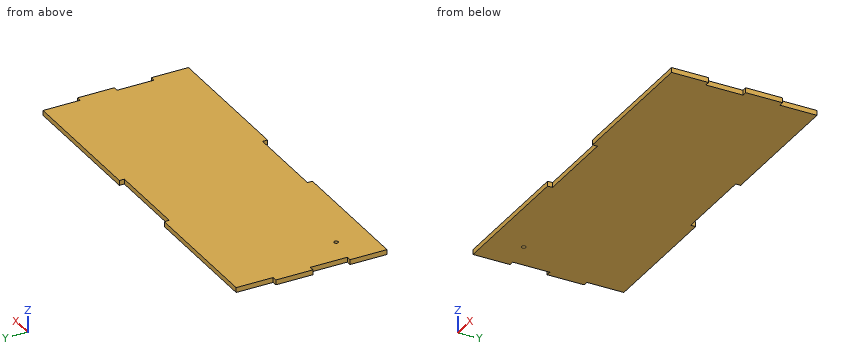
```python
from build123d import *

# Parameters (mm, degrees)
SKETCH1_R           = 1.25
BOSS_EXTRUDE1_DEPTH = 3


with BuildPart() as part:
    # Sketch1 → Boss-Extrude1 (new body)
    with BuildSketch(Plane.XY):
        Polygon((-2, 47), (78, 47), (78, 44), (128, 44), (128, 47), (213, 47), (213, 24.5), (216, 24.5), (216, 2), (213, 2), (213, -20.5), (216, -20.5), (216, -43), (213, -43), (128, -43), (128, -40), (78, -40), (78, -43), (-2, -43), (-5, -43), (-5, -20.5), (-2, -20.5), (-2, 2), (-5, 2), (-5, 24.5), (-2, 24.5), align=None)
        with Locations((15, -23)):
            Circle(SKETCH1_R, mode=Mode.SUBTRACT)
    extrude(amount=BOSS_EXTRUDE1_DEPTH)


solid = part.part
```
Check sheet for the modelled part. Datum: model origin and axes. Units: mm. Round coordinates to 2 decimals unless told otherwise and drop trailing zeros. Loops run counter-clockwise (first coordinate to the right, second up) from the corner with the lowest first, then second, coordinate; pieces in that order, holes last. Notation, with made-up numbers: (-9.75, -36.75) -> (35.25, -36.75) arc R20 ccw to (35.25, -16.75) -> close; hole circle Ø2 at (11.25, 40). An arc over 180 degrees is marked (long way). Write item = value, one per line. Start each with the question number.
1) Gauge pin test, flat ends, axial feed: pin 1 Ø0.9 at (y, z) = (45.5, 2) entering from -X; pin 2 Ø0.9 at (y, z) = (32, 1.5) entering from +X; pin 3 Ø0.9 at (x, z) = (215, 2) entering from +Y. Record the tip position at first contact, or that the pin passes through.
2) Thickness scan on probe 1 along Y at (x, z) = (15, 1.2); probe 2 along X at (y, z) = (26, 1.15); probe 3 along Y at (x, z) = (98, 1.8). Record the ranges inside material, lowest first.
3) Sectioned sample at A-A, the plane z = 2.3. Record the cut outline in (x, y), plus the area to 3 significant figures.
4) Sectioned sample at C-C, the plane x = 121. Record the cut outline in (y, z).
5) Sectioned sample at B-B, the plane y = -3.5. Record the cut outline in (x, z).
Results are:
q1.pin_1 = -2
q1.pin_2 = 213
q1.pin_3 = 24.5
q2.probe_1 = -43 to -24.25, -21.75 to 47
q2.probe_2 = -2 to 213
q2.probe_3 = -40 to 44
q3.outline = (-5, -43) -> (78, -43) -> (78, -40) -> (128, -40) -> (128, -43) -> (216, -43) -> (216, -20.5) -> (213, -20.5) -> (213, 2) -> (216, 2) -> (216, 24.5) -> (213, 24.5) -> (213, 47) -> (128, 47) -> (128, 44) -> (78, 44) -> (78, 47) -> (-2, 47) -> (-2, 24.5) -> (-5, 24.5) -> (-5, 2) -> (-2, 2) -> (-2, -20.5) -> (-5, -20.5) -> close; hole circle Ø2.5 at (15, -23)
q3.area = 19,300 mm^2
q4.outline = (-40, 0) -> (44, 0) -> (44, 3) -> (-40, 3) -> close
q5.outline = (-2, 0) -> (213, 0) -> (213, 3) -> (-2, 3) -> close
